Verification items for this drawing (mm, ordinates from the low corner). A direction names the side the tool comes from. Round coordinates to 2 decimals unless told otherwise and drop trailing zeros. Loops run counter-clockwise (first coordinate to the right, second up) from the corner with the lowest first, then second, coordinate; pieces in that order, holes last. Notation, with made-up numbers: (37, 15) - (72, 15) arc R27 ccw to (72, 52) - close; hole circle Ø2 at (89, 0.5). An arc over 180 degrees is marked (long way). Write item = value, one per line.
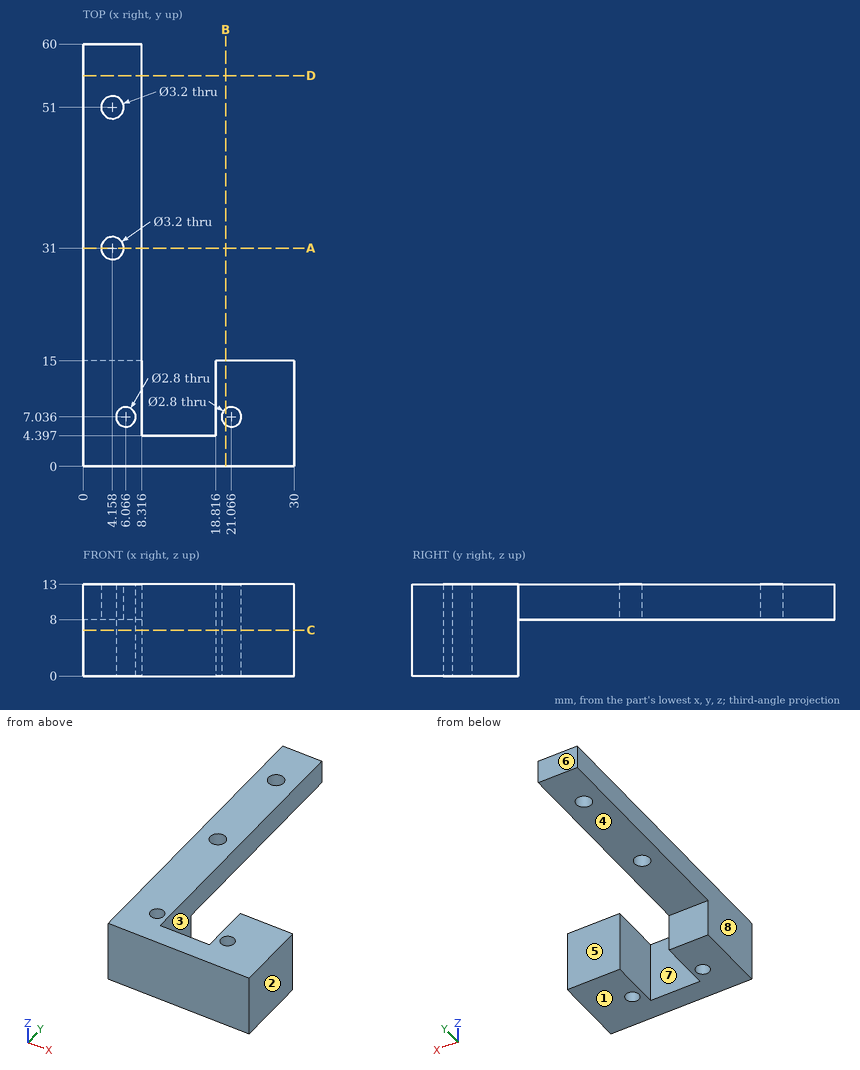
(1) Set-up check for the marked faces 4, 5, 6, 7 and 8: record each of +Z, -Z, +X, -X, +Y, -Y from which the full face is reachable in a straight line by a thin tool's end or side.
Answers follow:
face_4 = -Z, +X, -X, +Y
face_5 = +Z, -Z, +X, +Y
face_6 = +Z, -Z, +X, -X, +Y
face_7 = +Z, -Z, +Y
face_8 = +Z, -Z, -X, +Y, -Y
(2) Section check B-B (x = 20.25). Enter the section's corners in (y, z).
Answers follow:
outline = (0, 0) - (5.9, 0) - (5.9, 13) - (0, 13) - close; (8.17, 0) - (15, 0) - (15, 13) - (8.17, 13) - close
(3) Section check D-D (y = 55.5). Enter the section's corners in (x, z) (1 decimal), then the cut area to 3 significant figures.
Answers follow:
outline = (0, 8) - (8.3, 8) - (8.3, 13) - (0, 13) - close
area = 41.6 mm²
(4) Gauge pin test, flat ends, axial feed: pin 1 (1 mm diameter, centred on x = 24, z = 7, fed in from +Y); pin 2 (5 mm diameter, centred on x = 14, z = 9.5, fed in from +Y); pin 3 (3.5 mm diameter, centred on x = 21.07, y = 7.04, fed in from +Z); pin 4 (2.5 mm diameter, centred on x = 4, y = 34, fed in from -Z). Record the tip position at first contact, or that the pin passes through.
Answers follow:
pin_1 = 15
pin_2 = 4.4
pin_3 = 13
pin_4 = 8
(5) Section check A-A (y = 31). Enter the section's corners in (x, z) (1 decimal).
Answers follow:
outline = (0, 8) - (2.6, 8) - (2.6, 13) - (0, 13) - close; (5.8, 8) - (8.3, 8) - (8.3, 13) - (5.8, 13) - close
(6) Mould release check, pull along X, two halves, no side actions. Record for the marked faces 1, 2 and 3: pulls with the +X half, pulls with the -X half, needs draft (parallel to the pull), parting line crosses it, or undercut.
Answers follow:
face_1 = needs draft
face_2 = pulls with the +X half
face_3 = undercut
(7) Scan lines: L1, parallel to X at y = 12, z = 5.25 (1 decimal); L2, parallel to Y at x = 20.5, z = 8.25 (1 decimal); L3, parallel to Y at x = 18, z = 12.25. Record each from-to range of solid material in increasing order. Write a range as [from, to].
Answers follow:
L1 = [0, 8.3], [18.8, 30]
L2 = [0, 5.8], [8.3, 15]
L3 = [0, 4.4]
(8) Section check C-C (z = 6.5). Enter the section's corners in (x, y) (1 decimal).
Answers follow:
outline = (0, 0) - (30, 0) - (30, 15) - (18.8, 15) - (18.8, 4.4) - (8.3, 4.4) - (8.3, 15) - (0, 15) - close; hole circle Ø2.8 at (6.1, 7); hole circle Ø2.8 at (21.1, 7)
